Read the model definition and answer for the solid it produces. Units are mm, in the model's axes. A direction names the side the tool comes from. Give positions to 0.01 mm unless a question says otherwise; leave off trailing zeros. Loops run counter-clockwise (first coordinate to the right, second up) from the corner with the lowest first, then second, coordinate; pieces in that order, holes last. Notation, with made-up numbers: (-12, 9) -> (17, 9) arc R21 ccw to (17, 25) -> close; hole circle Ø8 at (32, 80.5). An arc over 180 degrees is marked (long way). Answer as CSV lines item,"result". Start each with the question number.
Autodesk Fusion 360 part; units mm, degrees
sketch "Sketch1" plane through (0, 0, 0) normal (0, 1, 0) x (1, 0, 0)
  line L0 (58.6438, 45) -> (-72.5, 45)
  line L1 (-72.5, 45) -> (-72.5, -45)
  line L2 (-72.5, -45) -> (58.6438, -45)
  line L3 (62.4739, 38.7769) -> (-72.5, -45) construction
  line L4 (-72.5, 45) -> (62.4739, -38.7769) construction
  line L5 (-72.5, 0) -> (-7.5, 0)
  arc A0 (58.6438, -45) -> (58.6438, 45) centre (-7.5, 0) ccw
  circle A1 centre (-7.5, 0) radius 23
  dimension "d2" = 90
  dimension "d3" = 65
  dimension "d4" = 160
  dimension "d7" = 46
extrude "Extrude2" add sketch "Sketch1" along normal blind 15 contours A1 makes body 1
extrude "Extrude1" add sketch "Sketch1" along normal blind 20 separate body contours A1 | L0 L1 L2 A0 makes body 2
combine "Combine1" operation cut target body 2 tool bodies 1
sketch "Sketch2" plane through (0, 20, 0) normal (0, 1, 0) x (-1, 0, 0)
  arc A0 (-58.6438, 45) -> (-58.6438, -45) centre (7.5, 0) ccw
  line L0 (-58.6438, -45) -> (72.5, -45)
  line L1 (72.5, -45) -> (72.5, 45)
  line L2 (72.5, 45) -> (-58.6438, 45)
  circle A1 centre (7.5, 0) radius 23
  circle A2 centre (7.5, 0) radius 30
  dimension "d10" = 60
extrude "Extrude3" add sketch "Sketch2" along normal blind 50 contours A1 | A2 bodies 2
sketch "Sketch3" plane through (0, 70, 0) normal (0, 1, 0) x (-1, 0, 0)
  circle A0 centre (7.5, 0) radius 30
  line L0 (7.5, -23) -> (27.4186, -11.5)
  line L1 (27.4186, -11.5) -> (27.4186, 11.5)
  line L2 (27.4186, 11.5) -> (7.5, 23)
  line L3 (7.5, 23) -> (-12.4186, 11.5)
  line L4 (-12.4186, 11.5) -> (-12.4186, -11.5)
  line L5 (-12.4186, -11.5) -> (7.5, -23)
  point P0 (7.5, 0)
  dimension "d13" = 23
extrude "Extrude4" cut sketch "Sketch3" against normal blind 55 contours L0 L1 L2 L3 L4 L5 bodies 2
ref_plane "WorkPlane1" through (-6.9281, 10, 45) normal (0, 0, 1) x (1, 0, 0)
sketch "Sketch4" plane through (-6.9281, 10, 45) normal (0, 0, 1) x (1, 0, 0)
  line L0 (29.4281, 60) -> (-30.5719, 60)
  line L1 (-30.5719, 10) -> (29.4281, 10)
  line L2 (-0.5719, 60) -> (-0.5719, 35)
  circle A0 centre (-0.5719, 35) radius 15
  dimension "d17" = 25
  dimension "d18" = 30
extrude "Extrude5" cut sketch "Sketch4" against normal blind 135 bodies 2
sketch "Sketch5" plane through (0, 20, 0) normal (0, 1, 0) x (-1, 0, 0)
  circle A0 centre (7.5, 0) radius 30
  arc A1 (-58.6438, 45) -> (-58.6438, -45) centre (7.5, 0) ccw
  line L0 (-58.6438, -45) -> (72.5, -45)
  line L1 (72.5, -45) -> (72.5, 45)
  line L2 (72.5, 45) -> (-58.6438, 45)
  line L3 (-47.5, -30) -> (62.5, -30)
  line L4 (62.5, -30) -> (62.5, 30)
  line L5 (62.5, 30) -> (-47.5, 30)
  line L6 (-47.5, 30) -> (-47.5, -30)
  line L7 (-47.5, -30) -> (62.5, 30) construction
  line L8 (62.5, -30) -> (-47.5, 30) construction
  line L9 (72.5, -45) -> (58.5, -45)
  line L10 (58.5, -45) -> (58.5, -30)
  line L11 (58.5, -30) -> (72.5, -30)
  line L12 (72.5, -30) -> (72.5, -45)
  circle A2 centre (-47.5, -30) radius 7
  circle A3 centre (-47.5, 30) radius 7
  circle A4 centre (58.5, -30) radius 8
  point P0 (7.5, 0)
  dimension "d21" = 110
  dimension "d22" = 60
  dimension "d23" = 14
  dimension "d24" = 15
  dimension "d25" = 14
  dimension "d26" = 14
  dimension "d27" = 16
extrude "Extrude6" cut sketch "Sketch5" against normal blind 20 contours L5 L6 A3 | L5 L6 A3 | L3 L6 A2 | L3 L6 A2 | L3 L4 L11 A4 | L3 L10 A4 | L4 L11 A4 | L3 L10 L11 A4 bodies 2
sketch "Sketch6" plane through (0, 20, 0) normal (0, 1, 0) x (-1, 0, 0)
  circle A0 centre (-47.5, 30) radius 7
  circle A1 centre (-47.5, -30) radius 7
  circle A2 centre (58.5, -30) radius 8
  circle A3 centre (7.5, 0) radius 30
  arc A4 (-58.6438, 45) -> (-58.6438, -45) centre (7.5, 0) ccw
  line L0 (-58.6438, -45) -> (72.5, -45)
  line L1 (72.5, -45) -> (72.5, 45)
  line L2 (72.5, 45) -> (-58.6438, 45)
  line L3 (58.5, -30) -> (58.5, 30) construction
  line L4 (72.5, 0) -> (58.5, 0) construction
  line L5 (58.5, -7) -> (79, -7)
  arc A5 (79, -7) -> (79, 7) centre (79, 0) ccw
  line L6 (79, 7) -> (58.5, 7)
  arc A6 (58.5, 7) -> (58.5, -7) centre (58.5, 0) ccw
  line L7 (58.5, 0) -> (79, 0) construction
  dimension "d30" = 14
extrude "Extrude7" cut sketch "Sketch6" against normal blind 5 contours L1 L5 L6 A6 bodies 2
sketch "Sketch7" plane through (0, 15, 0) normal (0, 1, 0) x (-1, 0, 0)
  arc A0 (58.5, 7) -> (58.5, -7) centre (58.5, 0) ccw
  line L0 (58.5, -7) -> (72.5, -7)
  line L1 (72.5, -7) -> (72.5, 7)
  line L2 (72.5, 7) -> (58.5, 7)
  line L3 (58.5, -4) -> (88, -4)
  arc A1 (88, -4) -> (88, 4) centre (88, 0) ccw
  line L4 (88, 4) -> (58.5, 4)
  arc A2 (58.5, 4) -> (58.5, -4) centre (58.5, 0) ccw
  line L5 (58.5, 0) -> (88, 0) construction
  dimension "d33" = 8
extrude "Extrude8" cut sketch "Sketch7" against normal blind 20 contours L1 L3 L4 A2 bodies 2
equation "d4 = ( 80 * 2 ) * 1 mm"
equation "d11 = 70 mm - 20 mm"
equation "d13 = ( 46 / 2 ) * 1 mm"
equation "d21 = ( 55 * 2 ) * 1 mm"
(1) A tool of negligible diameter and unlimited length cuts with its end or side. For faces 5 (the face through (-29, 15, 0)), 6 (the face through (12.419, 43, 0)), 7 (the face through (-65, 8, -4)), from which of +Z, -Z, +X, -X, +Y, -Y can it reach the whole face along a straight path? Write none if from no direction.
(2) Find section D-D on y = 36.5. Write down the section's boundary in (x, z).
(3) The mould has two halves that part along Y. Classify faces 1 (the face through (-22.485, 45.66, -22.046)), 2 (the face through (14, 15, 0)), 3 (the face through (-18.556, 55.138, 22.265)), 4 (the face through (-8, 10, 45)): pulls with the +Y half, pulls with the -Y half, needs draft (parallel to the pull), parting line crosses it, or undercut.
(4) Find section B-B on z = 0. Write down the section's boundary in (x, y), then the cut area to 3 significant figures.
(5) Find section A-A on y = 17. Write down the section's boundary in (x, z).
(6) Find section C-C on x = 47.5. Write down the section's boundary in (y, z).
(7) Each of these flat-tipped pins is pushed along its axis until it touches: P1, Ø7, axis at y = 46.5, z = 2, coming from the -X side; P2, Ø12.5, axis at x = -1.5, z = -14.5, coming from the -Y side; P3, Ø11, axis at x = -63, z = 1, coming from the +Y side. Where does it stop, or does it pass through?
(8) Find the intervals of material crossed by line 1 along Z through (x, y) = (47.5, 14.5); line 2 along Z through (x, y) = (-58, 10); line 3 along Y through (x, z) = (-7, -25), in increasing order. Write a range as from..to.
Answer block:
1,face 5,"-Y"
1,face 6,"+Y, -Y"
1,face 7,"-X, +Y, -Y"
2,outline,"(-27.42, -11.5) -> (-27.42, 11.5) -> (-19.86, 15.86) -> (-19.86, 27.34) arc R30 ccw to (-19.86, -27.34) -> (-19.86, -15.86) -> close; (4.86, -27.34) arc R30 ccw to (4.86, 27.34) -> (4.86, 15.86) -> (12.42, 11.5) -> (12.42, -11.5) -> (4.86, -15.86) -> close"
3,face 1,"undercut"
3,face 2,"pulls with the -Y half"
3,face 3,"undercut"
3,face 4,"needs draft"
4,outline,"(-54.5, 0) -> (-30.5, 0) -> (-30.5, 15) -> (-27.42, 15) -> (-27.42, 70) -> (-37.5, 70) -> (-37.5, 20) -> (-51.5, 20) -> (-51.5, 15) -> (-54.5, 15) -> close; (12.42, 15) -> (15.5, 15) -> (15.5, 0) -> (72.5, 0) -> (72.5, 20) -> (22.5, 20) -> (22.5, 70) -> (12.42, 70) -> close"
4,area,"2,640 mm2"
5,outline,"(-72.5, -45) -> (58.64, -45) arc R80 ccw to (58.64, 45) -> (-72.5, 45) -> (-72.5, 7) -> (-58.5, 7) arc R7 cw to (-58.5, -7) -> (-72.5, -7) -> close; hole circle Ø16 at (-58.5, -30); hole (-27.42, -11.5) -> (-7.5, -23) -> (12.42, -11.5) -> (12.42, 11.5) -> (-7.5, 23) -> (-27.42, 11.5) -> close; hole circle Ø14 at (47.5, -30); hole circle Ø14 at (47.5, 30)"
6,outline,"(0, -45) -> (20, -45) -> (20, -37) -> (0, -37) -> close; (0, -23) -> (20, -23) -> (20, 23) -> (0, 23) -> close; (0, 37) -> (20, 37) -> (20, 45) -> (0, 45) -> close"
7,P1,"stops at x = -37.5"
7,P2,"stops at y = 15"
7,P3,"stops at y = 15"
8,line 1,"z = -45..-37, -23..23, 37..45"
8,line 2,"z = -45..-37.98, -22.02..-3.97, 3.97..45"
8,line 3,"y = 0..30.01, 59.99..70"
